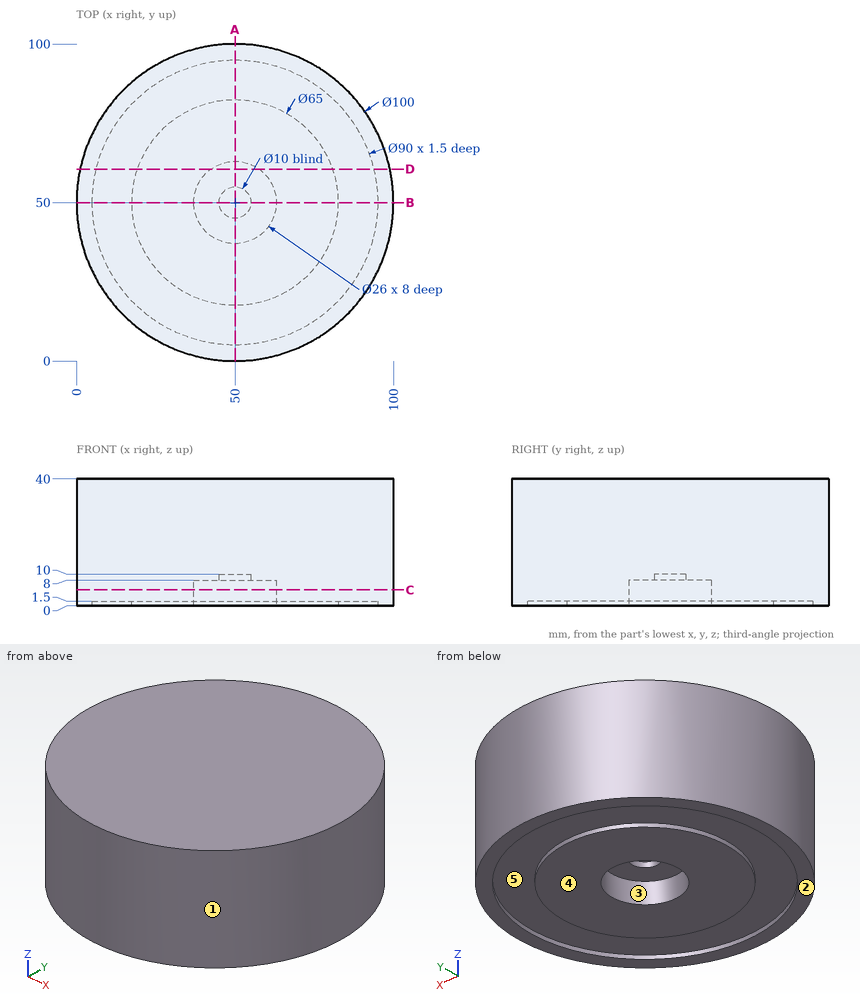
The drawing under review shows one solid part. Ordinate dimensions are in mm from its lowest x, y, z. A direction names the side the tool comes from. Give positions to 0.01 mm unless a question says otherwise; leave off trailing zeros. Write each loop counter-clockwise with the first axis right and the second up, starting at its lowest first coordinate (ties: lowest second). Pieces come first, ordered by that corner, then holes.
1. Add section D-D, the plane y = 60.5. Write out the cut boundary in (x, z), plus the area to 3 significant figures.
2. Tool access review of the marked faces 4 and 5: name each direction out of +Z, -Z, +X, -X, +Y, -Y from which nothing blocks a thin tool from reaching the whole face with its end or side.
3. Add section C-C, the plane z = 5. Write out the cut boundary in (x, y).
4. Add section A-A, the plane x = 50. Write out the cut boundary in (y, z).
5. Draft analysis for pull direction Y (two halves, no side actions). For the marked faces 1, 2 and 3, state which applies: +Y half, -Y half, draft (parallel to the pull), parting line (faces both ways), or undercut.
6. For P1, Ø4, axis at x = 50, y = 42, coming from the -Z side; P2, Ø5, axis at x = 51, y = 50, coming from the -Z side; P3, Ø10, axis at y = 32, z = 10.5, coming from the +X side, all flat-tipped, find the tip position at first contact; note any pin that passes through.
7. Wall thickness on L1, parallel to Y at x = 50, z = 9.55; L2, parallel to Y at x = 50, z = 4; L3, parallel to Z at x = 87, y = 51.5: over which ranges is each line inside the solid? List them lowest first.
Worked answers:
1. outline: (1.11, 0) - (6.24, 0) - (6.24, 1.5) - (19.24, 1.5) - (19.24, 0) - (42.34, 0) - (42.34, 8) - (57.66, 8) - (57.66, 0) - (80.76, 0) - (80.76, 1.5) - (93.76, 1.5) - (93.76, 0) - (98.89, 0) - (98.89, 40) - (1.11, 40) - close
1. area: 3,750 mm2
2. face 4: -Z, +X, -X, +Y, -Y
2. face 5: -Z
3. outline: circle Ø100 at (50, 50); hole circle Ø26 at (50, 50)
4. outline: (0, 0) - (5, 0) - (5, 1.5) - (17.5, 1.5) - (17.5, 0) - (37, 0) - (37, 8) - (45, 8) - (45, 10) - (55, 10) - (55, 8) - (63, 8) - (63, 0) - (82.5, 0) - (82.5, 1.5) - (95, 1.5) - (95, 0) - (100, 0) - (100, 40) - (0, 40) - close
5. face 1: parting line
5. face 2: draft
5. face 3: undercut
6. P1: stops at z = 8
6. P2: stops at z = 10
6. P3: stops at x = 98.28
7. L1: y = 0 to 45, 55 to 100
7. L2: y = 0 to 37, 63 to 100
7. L3: z = 1.5 to 40
